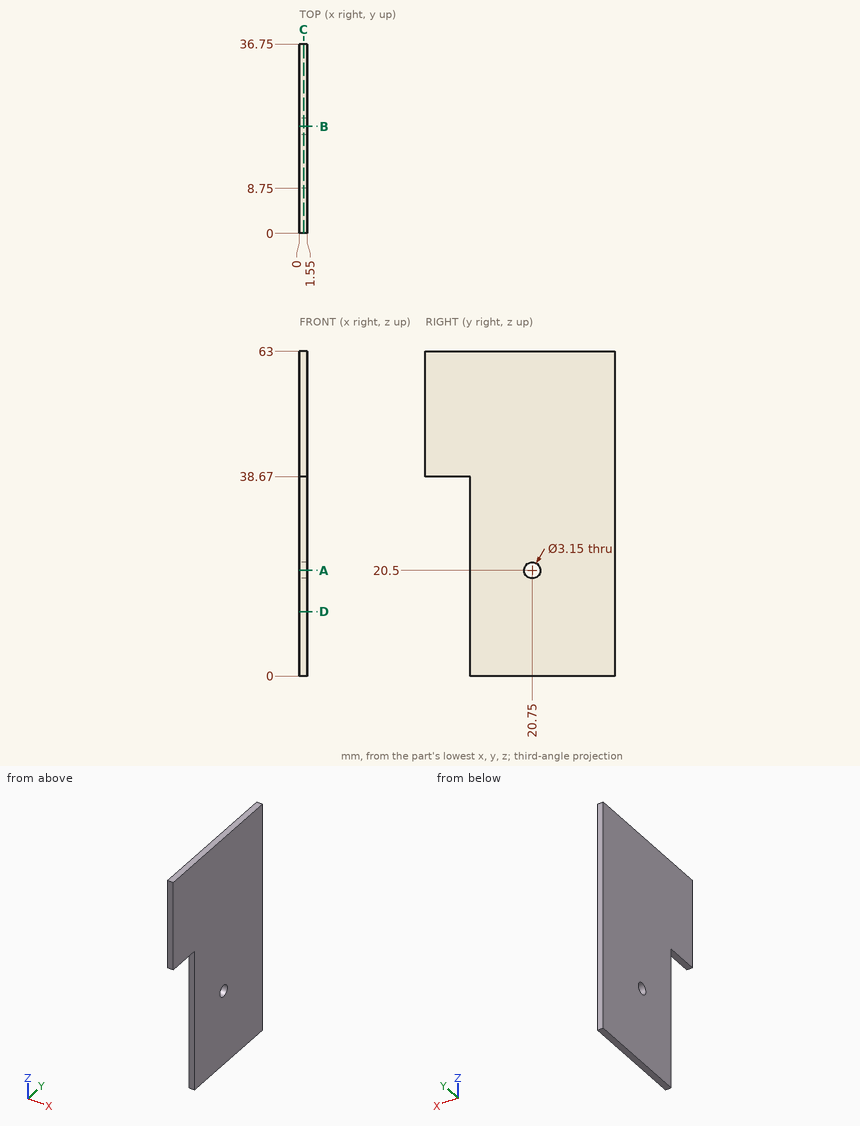
Can you work these out from the drawing? Everything is in mm from the part's minimum corner. Round coordinates to 2 decimals unless told otherwise and drop trailing zeros. Loops run counter-clockwise (first coordinate to the right, second up) from the corner with the lowest first, then second, coordinate; pieces in that order, holes last. Notation, with made-up numbers: (-39, 43) -> (-27, 43) arc R26 ccw to (-27, 74) -> close; hole circle Ø8 at (-34, -7). An arc over 180 degrees is marked (long way). Use CSV: the item, a comma, the result in double quotes.
(1) If I drill on probe 1 along Z at (x, y) = (0.6, 20.75) (3 decimals); probe 2 along Y at (x, z) = (0.6, 20.5) (3 decimals); probe 3 along Z at (x, y) = (0.95, 6.5), over which ranges is the centre line in solid material (lowest first)? Write a range as [from, to].
Return value:
probe 1,"z = [0, 18.925], [22.075, 63]"
probe 2,"y = [8.75, 19.175], [22.325, 36.75]"
probe 3,"z = [38.67, 63]"
(2) Suppose I cut it at B-B on y = 20.75. Write out the boundary of the cut face in (x, z) (3 decimals), plus the area to 3 significant figures.
Return value:
outline,"(0, 0) -> (1.55, 0) -> (1.55, 18.925) -> (0, 18.925) -> close; (0, 22.075) -> (1.55, 22.075) -> (1.55, 63) -> (0, 63) -> close"
area,"92.8 mm²"
(3) Suppose I cut it at C-C on x = 0.85. Write out the boundary of the cut face in (y, z) (3 decimals).
Return value:
outline,"(0, 38.67) -> (8.75, 38.67) -> (8.75, 0) -> (36.75, 0) -> (36.75, 63) -> (0, 63) -> close; hole circle Ø3.15 at (20.75, 20.5)"
(4) Suppose I cut it at D-D on z = 12.5. Write out the boundary of the cut face in (x, y), plus the area to 3 significant figures.
Return value:
outline,"(0, 8.75) -> (1.55, 8.75) -> (1.55, 36.75) -> (0, 36.75) -> close"
area,"43.4 mm²"
(5) Will this pin go through, and if not, where does the flat tip stop? pin 1 Ø0.5 at (x, z) = (1, 13) entering from -Y.
Return value:
pin 1,"stops at y = 8.75"
(6) Suppose I cut it at A-A on z = 20.5. Write out the boundary of the cut face in (x, y) (3 decimals), plus the area to 3 significant figures.
Return value:
outline,"(0, 8.75) -> (1.55, 8.75) -> (1.55, 19.175) -> (0, 19.175) -> close; (0, 22.325) -> (1.55, 22.325) -> (1.55, 36.75) -> (0, 36.75) -> close"
area,"38.5 mm²"
